Read the model definition and answer for the solid it produces. Units are mm, in the model's axes. Face numbers are marked on the shaded views. A direction names the side the tool comes from. Coordinates: 2 decimals unless noted, no trailing zeros. Order: outer loops, then holes, each group sorted by start corner. A loop starts at its lowest first (then second) coordinate and runs counter-clockwise, first axis right, second up. Notation, with made-up numbers: M -38,26 L -8,26 A26 cw -8,52 Z; hole C 88.5,39.5 d2. An arc over 180 degrees is marked long. Write each question's results on one line, items separated by ' | '.
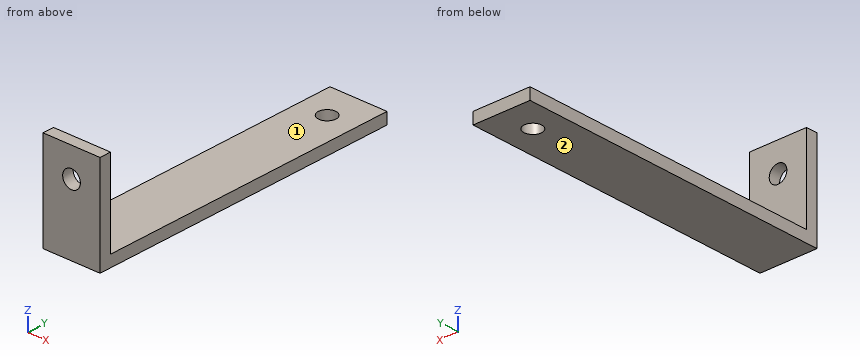
Autodesk Inventor part; units mm, degrees
ref_plane "YZ Plane" through (0, 0, 0) normal (1, 0, 0) x (0, 1, 0)
ref_plane "XZ Plane" through (0, 0, 0) normal (0, 1, 0) x (-1, 0, 0)
ref_plane "XY Plane" through (0, 0, 0) normal (0, 0, 1) x (1, 0, 0)
sketch "Sketch1" plane through (0, 0, 0) normal (0, 0, 1) x (1, 0, 0)
  line L0 (5, -2) -> (-5, -2)
  line L1 (5, -2) -> (5, 53)
  line L2 (5, 53) -> (-5, 53)
  line L3 (-5, 53) -> (-5, -2)
  line L4 (0, 53) -> (0, 47)
  circle A0 centre (0, 47) radius 1.55
  point P0 (0, 0)
  dimension "d3" = 2
  dimension "d16" = 55
  dimension "d17" = 10
  dimension "d18" = 6
  dimension "d19" = 3.1
extrude "Extrusion1" add sketch "Sketch1" against normal blind 2
sketch "Sketch2" plane through (0, 0, 0) normal (0, 0, 1) x (1, 0, 0)
  line L0 (-5, 0) -> (5, 0)
  line L1 (5, 0) -> (5, -2)
  line L2 (5, -2) -> (-5, -2)
  line L3 (-5, -2) -> (-5, 0)
  point P0 (0, 0)
extrude "Extrusion2" add sketch "Sketch2" along normal blind 15
sketch "Sketch3" plane through (-5, 0, 0) normal (0, 1, 0) x (1, 0, 0)
  circle A0 centre (5, -10) radius 1.55
  line L0 (10, -15) -> (0, -15)
  point P0 (5, 0)
  dimension "d11" = 3.1
  dimension "d15" = 5
extrude "Extrusion3" cut sketch "Sketch3" against normal blind 2
properties part number "spacer tutup"
(1) Given pin 1 (4 mm diameter, centred on x = -3.5, z = 7, fed in from +Y); pin 2 (3.5 mm diameter, centred on x = 0, y = 47, fed in from +Z), each flat-ended and moving along its own axis, determine where each tip first touches the part or whether it passes through.
Conclusion:
pin 1: y = 0 | pin 2: z = 0
(2) The part is cut by section B-B, the plane x = 0. Write down the section's boundary in (y, z).
Conclusion:
outline: M -2,-2 L 45.45,-2 L 45.45,0 L 0,0 L 0,8.45 L -2,8.45 Z; M -2,11.55 L 0,11.55 L 0,15 L -2,15 Z; M 48.55,-2 L 53,-2 L 53,0 L 48.55,0 Z
(3) The part is cut by section A-A, the plane y = 47. Write down the section's boundary in (x, z), then the cut area to 3 significant figures.
Conclusion:
outline: M -5,-2 L -1.55,-2 L -1.55,0 L -5,0 Z; M 1.55,-2 L 5,-2 L 5,0 L 1.55,0 Z | area: 13.8 mm²
(4) Straight lines are drawn through the part: line 1 (Y direction, x = 0, z = -0.8); line 2 (X direction, y = -0.75, z = 10); line 3 (Z direction, x = 0, y = -1.5). For each, find the intervals that lie inside material, in ascending order.
Conclusion:
line 1: -2 to 45.45, 48.55 to 53 | line 2: -5 to -1.55, 1.55 to 5 | line 3: -2 to 8.45, 11.55 to 15
(5) The part is cut by section D-D, the plane x = -2.5. Write down the section's boundary in (y, z), then the cut area to 3 significant figures.
Conclusion:
outline: M -2,-2 L 53,-2 L 53,0 L 0,0 L 0,15 L -2,15 Z | area: 140 mm²
(6) For the marked faces 1 and 2, determine the directions among +Z, -Z, +X, -X, +Y, -Y from which every point of the face is accessible in a straight line to the end or side of a thin tool.
Conclusion:
face 1: +Z, +X, -X, +Y | face 2: -Z, +X, -X, +Y, -Y
